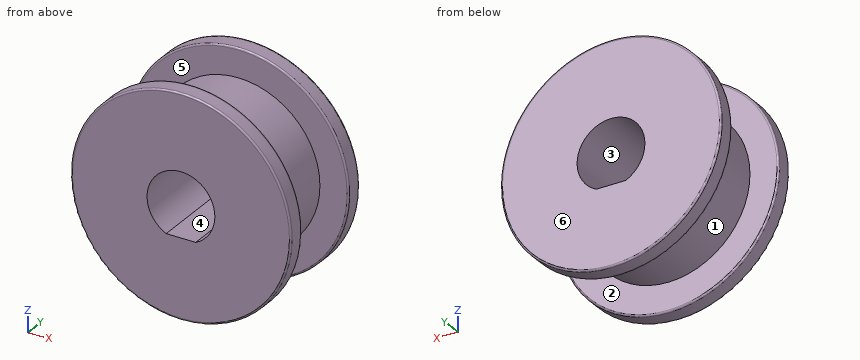
from build123d import *

# Parameters (mm, degrees)
SKETCH_2_R          = 6.5
EXTRUDE_1_DEPTH     = 6.5
SKETCH_4_R          = 6.5
SKETCH_4_R_2        = 4.8
CUT_EXTRUDE_1_DEPTH = 4.5
FILLET_1_R          = 0.1


with BuildPart() as part:
    # 草图2 → 凸台-拉伸1 (new body)
    with BuildSketch(Plane(origin=(0, 0, 0), x_dir=(1, 0, 0), z_dir=(0, 1, 0))):
        with Locations(Location((0, 0, 0), (0, 0, 90))):
            Circle(SKETCH_2_R)
        with BuildLine():
            Line((0.871779789, 1.8), (-0.871779789, 1.8))
            ThreePointArc((-0.871779789, 1.8), (0, -2), (0.871779789, 1.8))
        make_face(mode=Mode.SUBTRACT)
    extrude(amount=EXTRUDE_1_DEPTH)

    # 草图4 → 切除-拉伸1 (cut)
    with BuildSketch(Plane(origin=(0, 1, 0), x_dir=(-1, 0, 0), z_dir=(0, -1, 0))):
        with Locations(Location((0, 0, 0), (0, 0, 90))):
            Circle(SKETCH_4_R)
        with Locations(Location((0, 0, 0), (0, 0, 90))):
            Circle(SKETCH_4_R_2, mode=Mode.SUBTRACT)
    extrude(amount=-CUT_EXTRUDE_1_DEPTH, mode=Mode.SUBTRACT)

    # 圆角1
    fillet_1_edges = [part.edges().sort_by_distance(p)[0] for p in [
        (0, 5.5, 6.5),
        (0, 1, 6.5),
        (0, 0, 6.5),
        (0, 6.5, 6.5),
    ]]
    fillet(fillet_1_edges, radius=FILLET_1_R)


solid = part.part
Input: part model. Units: mm. Frame: model coordinates. Face numbers are marked on the shaded views. A direction names the side the tool comes from. Coordinates: 2 decimals unless noted, no trailing zeros. Loops run counter-clockwise (first coordinate to the right, second up) from the corner with the lowest first, then second, coordinate; pieces in that order, holes last.
(1) Section B-B on x = 0. Return the cut outline in (y, z).
(2) Section C-C on y = 4.5. Return the cut outline in (x, z).
(3) Set-up query: the marked faces 4, 5 and 6. Return all of +Z, -Z, +X, -X, +Y, -Y with unobstructed straight access to the full face (end or side cutting, diameter ignored); none if empty.
(4) Pull-direction query (X, two-part tool) for the marked faces 1, 2 and 3; classes: released by +X, released by -X, zero draft, split by the parting line, or undercut.
(5) Section A-A on z = 0. Return the cut outline in (x, y).
(6) Material intervals for probe 1 along X at (y, z) = (4, 0); probe 2 along Y at (x, z) = (-5.5, -1); probe 3 along X at (y, z) = (6.25, 0), sorted ascending.
(7) Section D-D on y = 6. Return the cut outline in (x, z), then the cut area to 3 significant figures.
(8) First-contact query: pin 1 Ø3 at (x, y) = (4, 1.5) entering from -Z; pin 2 Ø1 at (x, y) = (-3.5, 2) entering from +Z; pin 3 Ø3 at (y, z) = (5, 2.5) entering from +X. Flat tips, straight axial feed; report the tip coordinate or a pass-through.
Data:
1. outline: (0, -6.4) arc R0.1 ccw to (0.1, -6.5) - (0.9, -6.5) arc R0.1 ccw to (1, -6.4) - (1, -4.8) - (5.5, -4.8) - (5.5, -6.4) arc R0.1 ccw to (5.6, -6.5) - (6.4, -6.5) arc R0.1 ccw to (6.5, -6.4) - (6.5, -1.8) - (0, -1.8) - close; (0, 2) - (6.5, 2) - (6.5, 6.4) arc R0.1 ccw to (6.4, 6.5) - (5.6, 6.5) arc R0.1 ccw to (5.5, 6.4) - (5.5, 4.8) - (1, 4.8) - (1, 6.4) arc R0.1 ccw to (0.9, 6.5) - (0.1, 6.5) arc R0.1 ccw to (0, 6.4) - close
2. outline: circle Ø9.6 at (0, 0); hole (-0.87, -1.8) - (0.87, -1.8) arc R2 ccw (long way) to start
3. face 4: +Y, -Y
3. face 5: none
3. face 6: +Z, -Z, +X, -X, +Y
4. face 1: split by the parting line
4. face 2: zero draft
4. face 3: undercut
5. outline: (-6.5, 0.1) arc R0.1 ccw to (-6.4, 0) - (-2, 0) - (-2, 6.5) - (-6.4, 6.5) arc R0.1 ccw to (-6.5, 6.4) - (-6.5, 5.6) arc R0.1 ccw to (-6.4, 5.5) - (-4.8, 5.5) - (-4.8, 1) - (-6.4, 1) arc R0.1 ccw to (-6.5, 0.9) - close; (2, 0) - (6.4, 0) arc R0.1 ccw to (6.5, 0.1) - (6.5, 0.9) arc R0.1 ccw to (6.4, 1) - (4.8, 1) - (4.8, 5.5) - (6.4, 5.5) arc R0.1 ccw to (6.5, 5.6) - (6.5, 6.4) arc R0.1 ccw to (6.4, 6.5) - (2, 6.5) - close
6. probe 1: x = -4.8 to -2, 2 to 4.8
6. probe 2: y = 0 to 1, 5.5 to 6.5
6. probe 3: x = -6.5 to -2, 2 to 6.5
7. outline: circle Ø13 at (0, 0); hole (-0.87, -1.8) - (0.87, -1.8) arc R2 ccw (long way) to start
7. area: 120 mm2
8. pin 1: stops at z = -5.95
8. pin 2: stops at z = 3.75
8. pin 3: stops at x = 6.4
